Drawing for the job (mm, zero at the part's lowest x, y, z). A direction names the side the tool comes from. Coordinates: 2 decimals unless noted, no trailing zeros. One line per item, written item: value.
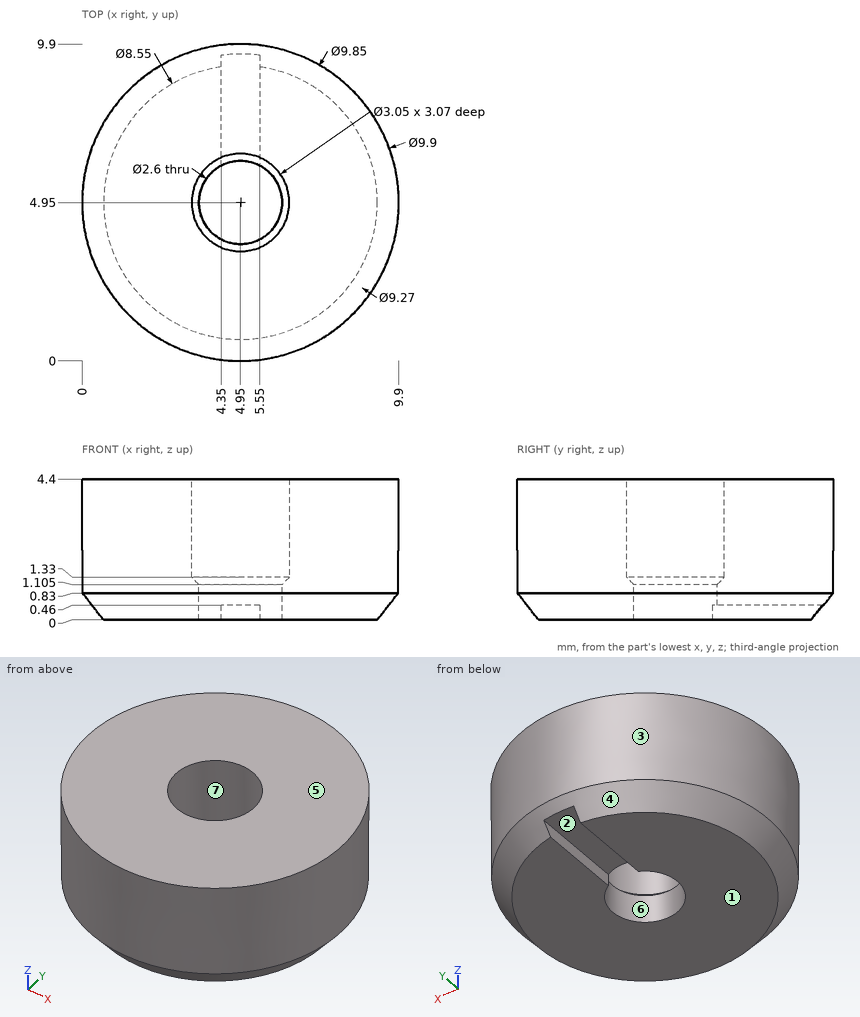
Item 1: Drop flat-ended pins along their axis: P1, Ø0.5, axis at y = 7.5, z = 0, coming from the -X side (1 decimal); P2, Ø1, axis at x = 5, y = 8.5, coming from the -Z side. Give the stop position or say it passes through.
Check result:
P1: stops at x = 1.2
P2: stops at z = 0.46
Item 2: Tool access for the marked faces 1, 2 and 3: list every direction of +Z, -Z, +X, -X, +Y, -Y with a clear straight run to the whole face (end or side of a thin tool).
Check result:
face 1: -Z, +X, -X, +Y, -Y
face 2: -Z, +Y
face 3: -Z
Item 3: Probe probe 1 along Y at (x, z) = (4.95, 2.75) (1 decimal); probe 2 along Y at (x, z) = (4.5, 0.5) (1 decimal); probe 3 along Y at (x, z) = (6.75, 1.45). List the from-to ranges inside material, lowest first. Write a range as from..to.
Check result:
probe 1: y = 0..3.4, 6.5..9.9
probe 2: y = 0.3..3.7, 6.2..9.6
probe 3: y = 0.36..9.54
Item 4: Pull direction X, two halves, no side cores. Call the marked faces 4, 5, 6 and 7: released by +X, released by -X, zero draft, split by the parting line, or undercut.
Check result:
face 4: split by the parting line
face 5: zero draft
face 6: undercut
face 7: undercut
